Build history of the part. All positions in model axes, mm. A direction names the side the tool comes from. Coordinates: 2 decimals unless noted, no trailing zeros. Order: outer loops, then holes, each group sorted by start corner. A loop starts at its lowest first (then second) coordinate and runs counter-clockwise, first axis right, second up. Notation, with made-up numbers: (70, 48.25) - (98, 48.25) arc R16 ccw to (98, 53.25) - close; hole circle Ø5 at (-20.75, 58). An arc over 180 degrees is marked (long way). Answer as CSV lines item,"result". Start each with the question number.
Solid Edge part; units mm, degrees
sketch "Sketch1" plane through (0, 0, 0) normal (0, 0, 1) x (1, 0, 0)
  circle A0 centre (0, 0) radius 4.25
extrude "Protrusion1" add sketch "Sketch1" along normal blind 5
sketch "Sketch2" plane through (0, 0, 5) normal (0, 0, 1) x (1, 0, 0)
  circle A0 centre (0, 0) radius 2.5
extrude "ExtrudedProtrusion_2" add sketch "Sketch2" along normal blind 20
sketch "Sketch3" plane through (0, 0, 0) normal (0, 0, -1) x (-1, 0, 0)
  line L0 (2.25, 0) -> (1.125, 1.9486)
  line L1 (1.125, 1.9486) -> (-1.125, 1.9486)
  line L2 (-1.125, 1.9486) -> (-2.25, 0)
  line L3 (-2.25, 0) -> (-1.125, -1.9486)
  line L4 (-1.125, -1.9486) -> (1.125, -1.9486)
  line L5 (1.125, -1.9486) -> (2.25, 0)
extrude "ExtrudedCutout_1" cut sketch "Sketch3" against normal blind 2.6
properties material "Stainless steel"
(1) Pull direction Y, two halves, no side cores. Call faces 1 (the flat face through (2, -1, 0)), 2 (the flat face through (-1.695, 0.961, 1.282)), 3 (the flat face through (0, 0, 2.6)), 4 (the cylindrical face through (2.285, -3.584, 2.465)): +Y half, -Y half, draft (parallel to the pull), parting line (faces both ways), or undercut.
(2) Band-saw the part on C-C on y = 2.25. List the corners of the cut face in (x, z).
(3) Band-saw the part on D-D on y = -0.25. List the corners of the cut face in (x, z).
(4) Band-saw the part on A-A on x = 0. List the corners of the cut face in (y, z).
(5) Drop flat-ended pins along their axis: pin 1 Ø1 at (x, z) = (1.5, 6.5) entering from +Y; pin 2 Ø0.7 at (x, z) = (0.5, 1.5) entering from +Y; pin 3 Ø1.2 at (x, y) = (-1, -0.5) entering from -Z. Give the stop position or say it passes through.
(6) Probe L1, parallel to Z at x = 3, y = 1; L2, parallel to Z at x = -0.75, y = -0.5; L3, parallel to Y at x = 0, z = 17.25. List the from-to ranges inside material, lowest first. Write a range as [from, to].
(7) Which spindle directions (+Z, -Z, +X, -X, +Y, -Y) get a long thin tool onto all of the face, cutting with end or side? Do faces 5 (the flat face through (0, 0, 25)), 6 (the cylindrical face through (-0.54, 2.44, 14.86)), 7 (the flat face through (0, 1.949, 1)). Say none if no direction does.
(8) Band-saw the part on B-B on z = 9.25. List the corners of the cut face in (x, y), plus the area to 3 significant figures.
Filled in:
1,face 1,"draft"
1,face 2,"undercut"
1,face 3,"undercut"
1,face 4,"parting line"
2,outline,"(-3.61, 0) - (3.61, 0) - (3.61, 5) - (1.09, 5) - (1.09, 25) - (-1.09, 25) - (-1.09, 5) - (-3.61, 5) - close"
3,outline,"(-4.24, 0) - (-2.11, 0) - (-2.11, 2.6) - (2.11, 2.6) - (2.11, 0) - (4.24, 0) - (4.24, 5) - (2.49, 5) - (2.49, 25) - (-2.49, 25) - (-2.49, 5) - (-4.24, 5) - close"
4,outline,"(-4.25, 0) - (-1.95, 0) - (-1.95, 2.6) - (1.95, 2.6) - (1.95, 0) - (4.25, 0) - (4.25, 5) - (2.5, 5) - (2.5, 25) - (-2.5, 25) - (-2.5, 5) - (-4.25, 5) - close"
5,pin 1,"stops at y = 2.29"
5,pin 2,"stops at y = 4.25"
5,pin 3,"stops at z = 2.6"
6,L1,"z = [0, 5]"
6,L2,"z = [2.6, 25]"
6,L3,"y = [-2.5, 2.5]"
7,face 5,"+Z, +X, -X, +Y, -Y"
7,face 6,"+Z"
7,face 7,"-Z"
8,outline,"circle Ø5 at (0, 0)"
8,area,"19.6 mm^2"
